Verification items for the finished model (mm, model axes). A direction names the side the tool comes from. Give positions to 0.01 mm unless a question says otherwise; leave off trailing zeros. Loops run counter-clockwise (first coordinate to the right, second up) from the corner with the lowest first, then second, coordinate; pieces in that order, holes last. Notation, with made-up numbers: (75.25, 9.5) - (113.25, 9.5) arc R27 cw to (113.25, 40.5) - close; hole circle Ø6 at (-30.5, 32.5). An arc over 180 degrees is marked (long way). Use one line per item in the form item = value.
```python
from build123d import *

# Parameters (mm, degrees)
SKETCH1_W                = 92
SKETCH1_H                = 70
SKETCH1_R                = 2.5
Y_PCB_EXTR_DEPTH         = 1.6
SKETCH2_W                = 31.5
SKETCH2_H                = 3.55
Y_HEADER_EXTR_DEPTH      = 8.5
SKETCH3_W                = 9.71
SKETCH3_H                = 62.95
SKETCH3_H_2              = 63.06
Y_MOLEX_POWER_EXTR_DEPTH = 12.88


with BuildPart() as part:
    # Sketch1 → Y+ PCB extr (new body)
    with BuildSketch(Plane(origin=(0, 0, 0), x_dir=(1, 0, 0), z_dir=(0, 1, 0))):
        with Locations((46, 35)):
            Rectangle(SKETCH1_W, SKETCH1_H)
        with Locations(Location((5.92, 3.07, 0), (0, 0, 270))):
            Circle(SKETCH1_R, mode=Mode.SUBTRACT)
        with Locations(Location((82.16, 3.07, 0), (0, 0, 270))):
            Circle(SKETCH1_R, mode=Mode.SUBTRACT)
        with Locations(Location((82.16, 67, 0), (0, 0, 270))):
            Circle(SKETCH1_R, mode=Mode.SUBTRACT)
        with Locations(Location((5.92, 67, 0), (0, 0, 270))):
            Circle(SKETCH1_R, mode=Mode.SUBTRACT)
    extrude(amount=Y_PCB_EXTR_DEPTH)

    # Sketch2 → Y+ header extr (add)
    with BuildSketch(Plane(origin=(0, 1.6, 0), x_dir=(1, 0, 0), z_dir=(0, 1, 0))):
        with Locations((45.7, 66.165)):
            Rectangle(SKETCH2_W, SKETCH2_H)
    extrude(amount=Y_HEADER_EXTR_DEPTH)

    # Sketch3 → Y- MOLEX power extr (add)
    with BuildSketch(Plane.XZ):
        with Locations((73.775, -33.605)):
            Rectangle(SKETCH3_W, SKETCH3_H)
        with Locations((17.735, -33.66)):
            Rectangle(SKETCH3_W, SKETCH3_H_2)
    extrude(amount=Y_MOLEX_POWER_EXTR_DEPTH)


solid = part.part
```
1. Section check D-D, the plane z = -31.5. Record the cut outline in (x, y).
Result set:
outline = (0, 0) - (12.88, 0) - (12.88, -12.88) - (22.59, -12.88) - (22.59, 0) - (68.92, 0) - (68.92, -12.88) - (78.63, -12.88) - (78.63, 0) - (92, 0) - (92, 1.6) - (0, 1.6) - close
2. Section check B-B, the plane y = -7.75. Record the cut outline in (x, z), then the cut area to 3 significant figures.
Result set:
outline = (12.88, -65.19) - (22.59, -65.19) - (22.59, -2.13) - (12.88, -2.13) - close; (68.92, -65.08) - (78.63, -65.08) - (78.63, -2.13) - (68.92, -2.13) - close
area = 1,220 mm²
3. Section check A-A, the plane x = 5.92. Record the cut outline in (y, z).
Result set:
outline = (0, -70) - (1.6, -70) - (1.6, -69.5) - (0, -69.5) - close; (0, -64.5) - (1.6, -64.5) - (1.6, -5.57) - (0, -5.57) - close; (0, -0.57) - (1.6, -0.57) - (1.6, 0) - (0, 0) - close
4. Tool access check on faces 5 (the flat face through (61.45, 6, -66)), 6 (the flat face through (45, 6, -67.94)), 7 (the flat face through (74, -6, -2.13)), 8 (the flat face through (22.59, -6, -34)), 9 (the flat face through (18, -6, -65.19)). Record the directions out of +Z, -Z, +X, -X, +Y, -Y that give a thin tool (end or side, any length) a straight path to the whole face; none if there is none.
Result set:
face_5 = +Z, -Z, +X, +Y
face_6 = -Z, +X, -X, +Y
face_7 = +Z, +X, -X, -Y
face_8 = +Z, -Z, -Y
face_9 = -Z, +X, -X, -Y
5. Depth check by flat-ended pin: pin 1 Ø4 at (x, y) = (44.5, 4.5) entering from +Z; pin 2 Ø4 at (y, z) = (4.5, -66.5) entering from +X; pin 3 Ø3 at (x, z) = (5.92, -3.07) entering from +Y; pin 4 Ø5 at (x, y) = (16, -8) entering from +Z. Enter the tip coordinate at first touch or a pass-through.
Result set:
pin_1 = -64.39
pin_2 = 61.45
pin_3 = through
pin_4 = -2.13
6. Scan lines: probe 1 along X at (y, z) = (-2.5, -11); probe 2 along X at (y, z) = (0.8, -67); probe 3 along Z at (x, y) = (61, 7.75). Record each from-to range of solid material in increasing order.
Result set:
probe_1 = 12.88 to 22.59, 68.92 to 78.63
probe_2 = 0 to 3.42, 8.42 to 79.66, 84.66 to 92
probe_3 = -67.94 to -64.39
7. Section check C-C, the plane x = 57. Record the cut outline in (y, z), then the cut area to 3 significant figures.
Result set:
outline = (0, -70) - (1.6, -70) - (1.6, -67.94) - (10.1, -67.94) - (10.1, -64.39) - (1.6, -64.39) - (1.6, 0) - (0, 0) - close
area = 142 mm²
8. Draft check along X on faces 1 (the cylindrical face through (8.4, 0.8, -3.4)), 2 (the flat face through (78.63, -6, -34)), 3 (the cylindrical face through (79.72, 0.79, -3.61)), 4 (the flat face through (45, 6, -64.39)). Enter one of: released by +X, released by -X, zero draft, split by the parting line, or undercut.
Result set:
face_1 = undercut
face_2 = released by +X
face_3 = undercut
face_4 = zero draft
